Build history of the part. All positions in model axes, mm. Round coordinates to 2 decimals unless told otherwise and drop trailing zeros. Order: outer loops, then holes, each group sorted by start corner. A loop starts at its lowest first (then second) coordinate and runs counter-clockwise, first axis right, second up. Notation, with made-up numbers: (-16.5, -11.75) -> (22.5, -11.75) arc R24 cw to (22.5, -0.75) -> close; hole circle Ø3 at (44.5, 56). An arc over 180 degrees is marked (long way). Use a Markdown table: item, result. Add a question column.
Item 1: Pin check, flat tips, straight feed: pin 1 (12 mm diameter, centred on x = -13, y = -19, fed in from -Z); pin 2 (1 mm diameter, centred on x = -3, y = -37.5, fed in from +Z); pin 3 (1.5 mm diameter, centred on y = -10.5, z = 2, fed in from +X). Stop position of each tip, or through.
Item 2: Slice it at C-C, the plane y = -6.5. Give the cut face in (x, z).
Item 3: Slice it at D-D, the plane y = -38. Give the cut face in (x, z), plus the area to 3 significant figures.
Item 4: Two-plate mould, pull along Z, no slides. Class faces 1 (the face through (1.38, -4.68, 6.2)), 2 (the face through (12.932, -7.571, -5.362)), 3 (the face through (3, 0, -6)): released by +Z, released by -Z, zero draft, split by the parting line, or undercut.
Item 5: Probe L1, parallel to Z at x = 0, y = -4; L2, parallel to X at y = -15, z = -9; L3, parallel to Y at x = 5.5, z = 7. List the from-to ranges inside material, lowest first.
Item 6: Slice it at B-B, the plane z = 0. Give the cut face in (x, y), plus the area to 3 significant figures.
Item 7: Slice it at A-A, the plane x = 0. Give the cut face in (y, z).
from build123d import *

# Parameters (mm, degrees)
F0_R     = 14
F0_R_2   = 11.6
F1_DEPTH = 25
F2_D     = 12.7
F2_DEPTH = 14
F2_TIP   = 3.8154649308


# Not quite as in the source:
# - a length typed as a fraction of an inch, garbled in the dataset ("3 / 203.2 mm" for 3/8 in), is restored


with BuildPart() as f1:
    # F0 (on Front) → F1 (new body)
    with BuildSketch(Plane.XZ):
        Circle(F0_R)
        Circle(F0_R_2, mode=Mode.SUBTRACT)
        Circle(F0_R_2)
    extrude(amount=F1_DEPTH)

    # F2
    with Locations(Plane(origin=(0, 0, 0), x_dir=(1, 0, 0), z_dir=(0, 1, 0))):
        with Locations((0, 0)):
            Hole(F2_D / 2, depth=F2_DEPTH)
            with Locations((0, 0, -(F2_DEPTH + F2_TIP / 2))):  # 118° drill point
                Cone(0, F2_D / 2, F2_TIP, mode=Mode.SUBTRACT)

    # F3 (on face) → F4 (revolve)
    with BuildSketch(Plane.XZ.offset(25)):
        with BuildLine():
            Line((17, 0), (14, 0))
            ThreePointArc((14, 0), (0, -14), (-14, 0))
            Line((-14, 0), (-17, 0))
            ThreePointArc((-17, 0), (0, -17), (17, 0))
        make_face()
        with BuildLine():
            ThreePointArc((-14, 0), (0, -14), (14, 0))
            Line((14, 0), (-14, 0))
        make_face()
    revolve(axis=Axis((0, -25, 0), (1, 0, 0)))


solid = f1.part
Check sheet entries:
| question | item | result |
|---|---|---|
| 1 | pin 1 | z = -14.83 |
| 1 | pin 2 | z = 11.68 |
| 1 | pin 3 | x = 13.94 |
| 2 | outline | circle Ø28 at (0, 0); hole circle Ø12.7 at (0, 0) |
| 3 | outline | circle Ø21.91 at (0, 0) |
| 3 | area | 377 mm2 |
| 4 | face 1 | undercut |
| 4 | face 2 | split by the parting line |
| 4 | face 3 | zero draft |
| 5 | L1 | -14 to -6.35, 6.35 to 14 |
| 5 | L2 | -10.72 to 10.72 |
| 5 | L3 | -39.48 to 0 |
| 6 | outline | (-14, -15.36) arc R17 ccw (long way) to (14, -15.36) -> (14, 0) -> (6.35, 0) -> (6.35, -9.23) arc R17 ccw to (-6.35, -9.23) -> (-6.35, 0) -> (-14, 0) -> close |
| 6 | area | 1,090 mm2 |
| 7 | outline | (-15.36, -14) -> (0, -14) -> (0, -6.35) -> (-9.23, -6.35) arc R17 ccw to (-9.23, 6.35) -> (0, 6.35) -> (0, 14) -> (-15.36, 14) arc R17 ccw (long way) to start |
